The listing builds one solid part. Answer for the finished solid, in the listing's coordinates (mm). Face numbers are marked on the shaded views. A direction names the side the tool comes from. Round coordinates to 2 decimals unless told otherwise and drop trailing zeros. Write each loop counter-clockwise with the first axis right and the second up, starting at its lowest first coordinate (ties: lowest second). Pieces come first, ordered by that corner, then holes. Notation, with made-up numbers: (81.5, -8.75) - (112.5, -8.75) arc R14 cw to (112.5, 9.25) - close; hole circle Ø1 at (72.5, 14). An arc over 180 degrees is marked (long way). Use a Markdown table: item, result. Add a question column.
1) Determine the mould class of the marked faces 1, 2, 3 and 4 for opening direction X: +X half, -X half, draft (parallel to the pull), parting line (faces both ways), or undercut.
2) A cutting plane is placed at A-A (x = -12.5). Give the vertices of the cut face in (y, z), then the cut area to 3 significant figures.
3) A cutting plane is placed at B-B (y = 10). Give the vertices of the cut face in (x, z), then the cut area to 3 significant figures.
4) A cutting plane is placed at C-C (z = 0). Give the vertices of the cut face in (x, y), then the cut area to 3 significant figures.
5) Find the intervals of material crossed by probe 1 along X at (y, z) = (3, 0); probe 2 along X at (y, z) = (2, 2.5); probe 3 along Z at (x, y) = (12.5, 1.8), in increasing order. Write a range as from..to.
6) Each of these flat-tipped pins is pushed along its axis until it touches: P1, Ø4.5, axis at x = -14, z = -1, coming from the +Y side; P2, Ø5, axis at y = 10.5, z = 1.5, coming from the -X side. Where does it stop, or does it pass through?
7) A tool of negligible diameter and unlimited length cuts with its end or side. For the marked faces 5 and 6, from which of +Z, -Z, +X, -X, +Y, -Y can it reach the whole face along a straight path? Write none if from no direction.
8) A cutting plane is placed at D-D (z = 5). Give the vertices of the cut face in (x, y).
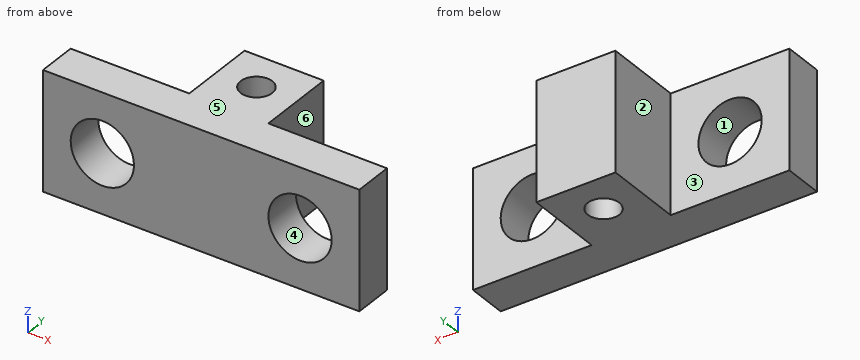
```python
from build123d import *

# Parameters (mm, degrees)
SKETCH_1_W          = 40
SKETCH_1_H          = 15
EXTRUDE_3_DEPTH     = 5
SKETCH_2_W          = 10
SKETCH_2_H          = 15
EXTRUDE_4_DEPTH     = 10
SKETCH_4_R          = 2
CUT_EXTRUDE_1_DEPTH = 30.154759474
SKETCH_8_R          = 4
CUT_EXTRUDE_3_DEPTH = 24.58495283


with BuildPart() as part:
    # 草图1 → 凸台-拉伸3 (new body)
    with BuildSketch(Plane(origin=(0, 0, 0), x_dir=(1, 0, 0), z_dir=(0, 1, 0))):
        Rectangle(SKETCH_1_W, SKETCH_1_H)
    extrude(amount=EXTRUDE_3_DEPTH)

    # 草图2 → 凸台-拉伸4 (add)
    with BuildSketch(Plane(origin=(0, 5, 0), x_dir=(1, 0, 0), z_dir=(0, 1, 0))):
        Rectangle(SKETCH_2_W, SKETCH_2_H)
    extrude(amount=EXTRUDE_4_DEPTH)

    # 草图4 → 切除-拉伸1 (cut, through all)
    with BuildSketch(Plane(origin=(0, 0, -7.5), x_dir=(-1, 0, 0), z_dir=(0, 0, -1))):
        with Locations((0, 10)):
            Circle(SKETCH_4_R)
    extrude(amount=-CUT_EXTRUDE_1_DEPTH, mode=Mode.SUBTRACT)

    # 草图8 → 切除-拉伸3 (cut, through all)
    with BuildSketch(Plane(origin=(0, 5, 0), x_dir=(1, 0, 0), z_dir=(0, 1, 0))):
        with Locations(Location((-12.5, 0, 0), (0, 0, 270))):
            Circle(SKETCH_8_R)
    cut_extrude_3 = extrude(amount=-CUT_EXTRUDE_3_DEPTH, mode=Mode.SUBTRACT)

    # 镜向1: 切除-拉伸3 across plane
    add(cut_extrude_3.mirror(Plane(origin=(0, 0, 0), x_dir=(0, 0, 1), z_dir=(1, 0, 0))), mode=Mode.SUBTRACT)


solid = part.part
```
Entries:
| question | item | result |
|---|---|---|
| 1 | face 1 | undercut |
| 1 | face 2 | -X half |
| 1 | face 3 | draft |
| 1 | face 4 | undercut |
| 2 | outline | (0, -7.5) - (5, -7.5) - (5, -4) - (0, -4) - close; (0, 4) - (5, 4) - (5, 7.5) - (0, 7.5) - close |
| 2 | area | 35.0 mm² |
| 3 | outline | (-5, -7.5) - (-2, -7.5) - (-2, 7.5) - (-5, 7.5) - close; (2, -7.5) - (5, -7.5) - (5, 7.5) - (2, 7.5) - close |
| 3 | area | 90.0 mm² |
| 4 | outline | (-20, 0) - (-16.5, 0) - (-16.5, 5) - (-20, 5) - close; (-8.5, 0) - (8.5, 0) - (8.5, 5) - (5, 5) - (5, 15) - (-5, 15) - (-5, 5) - (-8.5, 5) - close; (16.5, 0) - (20, 0) - (20, 5) - (16.5, 5) - close; hole circle Ø4 at (0, 10) |
| 4 | area | 207 mm² |
| 5 | probe 1 | x = -20..-16.5, -8.5..8.5, 16.5..20 |
| 5 | probe 2 | x = -20..-15.62, -9.38..9.38, 15.62..20 |
| 5 | probe 3 | z = -7.5..-4, 4..7.5 |
| 6 | P1 | stops at y = 5 |
| 6 | P2 | stops at x = -5 |
| 7 | face 5 | +Z, +X, -X, +Y, -Y |
| 7 | face 6 | +Z, -Z, +X, +Y |
| 8 | outline | (-20, 0) - (20, 0) - (20, 5) - (5, 5) - (5, 15) - (-5, 15) - (-5, 5) - (-20, 5) - close; hole circle Ø4 at (0, 10) |
